The drawing under review shows one solid part. Ordinate dimensions are in mm from its lowest x, y, z. A direction names the side the tool comes from. Coordinates: 2 decimals unless noted, no trailing zeros. Order: outer loops, then holes, each group sorted by start corner. A loop starts at its lowest first (then second) coordinate and runs counter-clockwise, first axis right, second up.
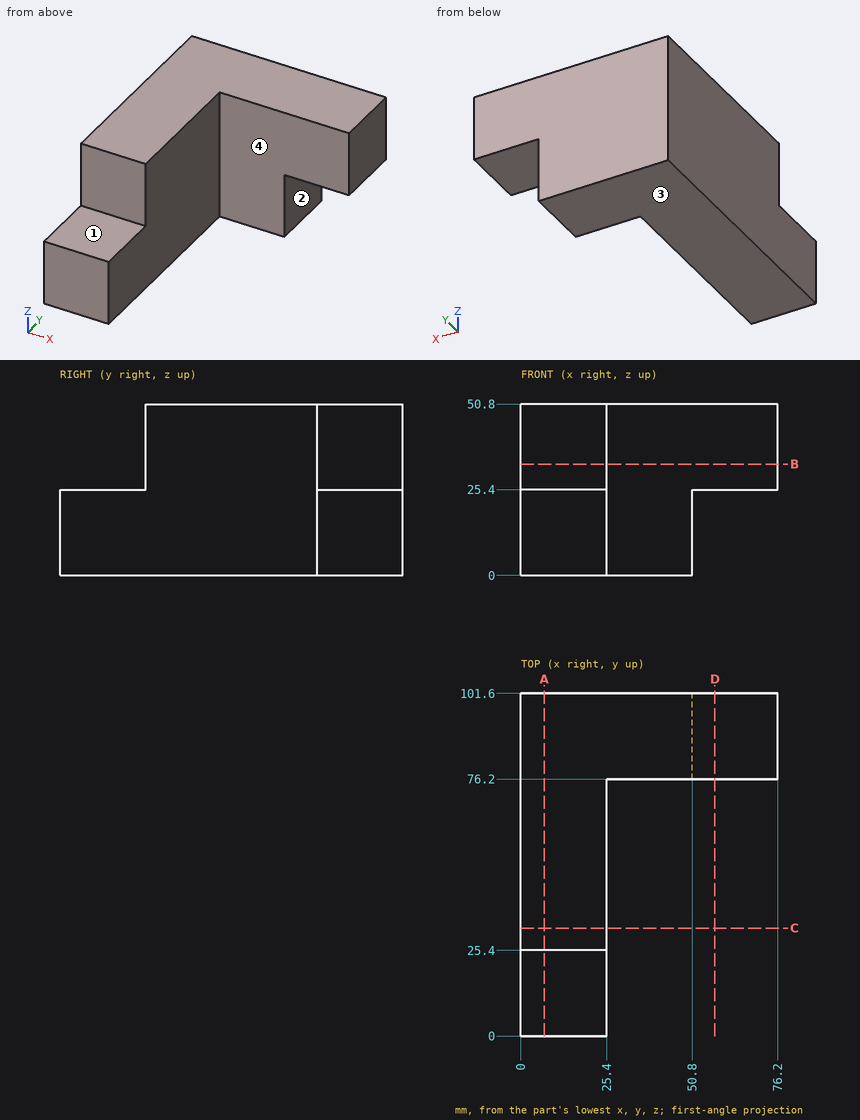
1. Take a section at B-B, the plane z = 33. Give the boundary of the cut face in (x, y), plus the area to 3 significant figures.
Answer below:
outline: (0, 25.4) - (25.4, 25.4) - (25.4, 76.2) - (76.2, 76.2) - (76.2, 101.6) - (0, 101.6) - close
area: 3,230 mm2
2. Take a section at A-A, the plane x = 7. Give the boundary of the cut face in (y, z).
Answer below:
outline: (0, 0) - (101.6, 0) - (101.6, 50.8) - (25.4, 50.8) - (25.4, 25.4) - (0, 25.4) - close
3. Clearance check with flat-ended pins moving along their axes: pin 1 Ø3 at (y, z) = (38, 23.5) entering from +X; pin 2 Ø12 at (x, z) = (53.5, 40) entering from -Y; pin 3 Ø12.5 at (x, y) = (14, 14.5) entering from +Z. State where each tip first meets the part, or that it passes through.
Answer below:
pin 1: stops at x = 25.4
pin 2: stops at y = 76.2
pin 3: stops at z = 25.4
4. Take a section at D-D, the plane x = 57.5. Give the boundary of the cut face in (y, z), plus the area to 3 significant figures.
Answer below:
outline: (76.2, 25.4) - (101.6, 25.4) - (101.6, 50.8) - (76.2, 50.8) - close
area: 645 mm2
5. Machinability: for the marked faces 1, 2, 3 and 4, which of the approach directions +Z, -Z, +X, -X, +Y, -Y give a long, thin tool a straight path to every point of the face, cutting with its end or side? Answer none if there is none.
Answer below:
face 1: +Z, +X, -X, -Y
face 2: -Z, +X, +Y, -Y
face 3: -Z, +X, -X, +Y, -Y
face 4: +Z, -Z, +X, -Y
6. Take a section at C-C, the plane y = 32. Give the boundary of the cut face in (x, z), plus the area to 3 significant figures.
Answer below:
outline: (0, 0) - (25.4, 0) - (25.4, 50.8) - (0, 50.8) - close
area: 1,290 mm2
7. To check wall thickness, follow L1, parallel to Y at x = 21.5, z = 32.5; L2, parallel to X at y = 31, z = 8. State the ranges of each line that lie inside material, in increasing order.
Answer below:
L1: y = 25.4 to 101.6
L2: x = 0 to 25.4
